Drawing for the job (mm, zero at the part's lowest x, y, z). Give positions to 0.01 mm unless a question says otherwise; leave off trailing zeros. Loops run counter-clockwise (first coordinate to the right, second up) from the corner with the lowest first, then second, coordinate; pieces in that order, holes last.
1) Wall check: line 1 (Z direction, x = 509, y = 2); line 2 (X direction, y = 7.75, z = 109) (1 decimal); line 3 (X direction, y = 11.5, z = 56). Give the ranges that are in metal, low to high.
2) Flat gauge pins, fed straight in: P1, Ø2, axis at x = 108.5, y = 5.5, coming from the +Z side; P2, Ø1, axis at y = 12.5, z = 23, coming from the +X side; P3, Ø10, axis at y = 9.5, z = 110, coming from the +X side. Where does each tip first touch, or does it go through?
3) Band-saw the part on B-B on x = 103. List the corners of the cut face in (y, z), then the cut area to 3 significant figures.
4) Band-saw the part on C-C on z = 106. List the corners of the cut face in (x, y).
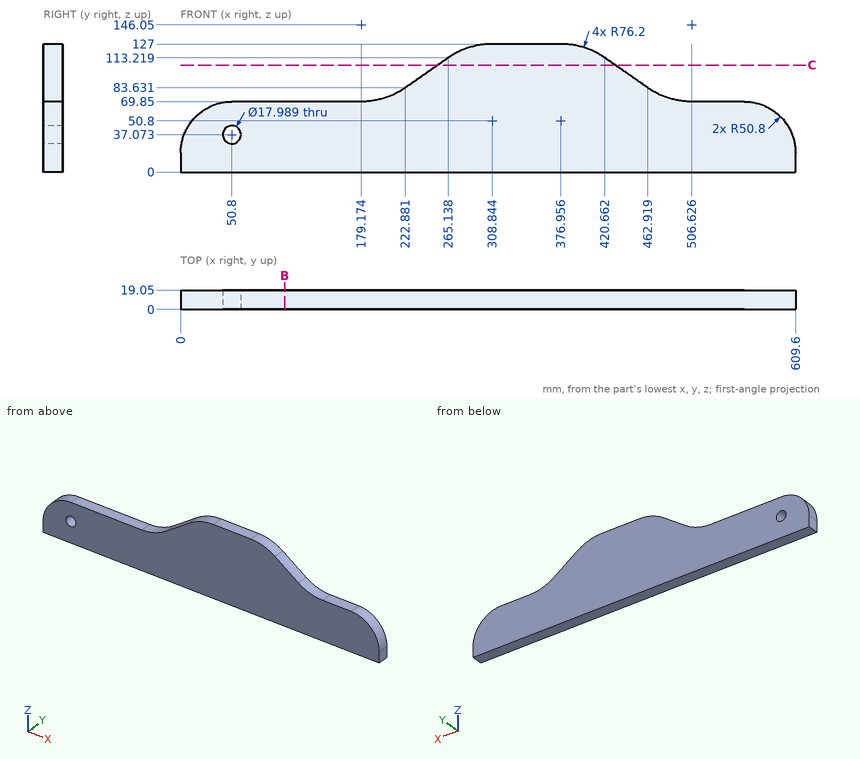
Findings below:
1. line 1: z = 0 to 69.85
1. line 2: x = 259.1 to 426.7
1. line 3: x = 15.94 to 593.66
2. P1: stops at z = 69.85
2. P2: stops at x = 609.48
2. P3: stops at x = 432.4
3. outline: (0, 0) - (19.05, 0) - (19.05, 69.85) - (0, 69.85) - close
3. area: 1,330 mm2
4. outline: (254.83, 0) - (430.97, 0) - (430.97, 19.05) - (254.83, 19.05) - close
